Could you check a few things on this model? Use its own coordinates, in mm. Face numbers are marked on the shaded views. Give positions to 0.01 mm unless a question says otherwise; leave off trailing zeros. Write each loop counter-clockwise with the first axis right and the second up, starting at its lowest first coordinate (ties: lowest second). Pieces come first, ordered by that corner, then holes. Notation, with made-up numbers: (58, -15.75) - (108, -15.75) arc R27 cw to (108, 1.25) - close; hole circle Ø1 at (2, 20.25). An arc over 180 degrees is marked (long way). Answer in a Markdown table with one row per item.
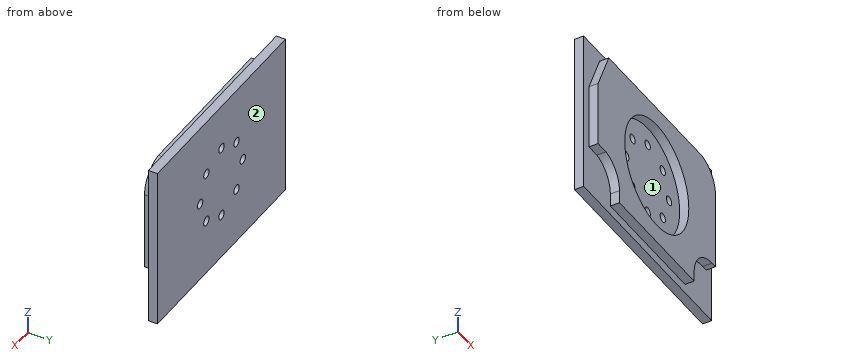
from build123d import *

# Parameters (mm, degrees)
F0_W     = 120
F0_H     = 90
F1_DEPTH = 5
F3_D     = 5
F4_R     = 2.5
F5_DEPTH = 5
F6_R     = 30
F7_DEPTH = 5


with BuildPart() as f1:
    # F0 (on Front) → F1 (new body)
    with BuildSketch(Plane.XZ):
        with Locations((-60, 45)):
            Rectangle(F0_W, F0_H)
    extrude(amount=F1_DEPTH)

    # F3 (through all)
    with Locations(Plane.XZ.offset(5)):
        with Locations((-74.144270925, 59.14), (-60, 65), (-45.86, 59.144270925), (-40, 45), (-45.855729075, 30.86), (-60, 25), (-80, 45), (-74.144270925, 30.86)):
            Hole(F3_D / 2)

    # F4 (on face) → F5 (join)
    with BuildSketch(Plane.XZ.offset(5)):
        with BuildLine():
            Line((-5, 27), (-5, 70.1358293132))
            ThreePointArc((-5, 70.1358293132), (-8.7037424203, 80.0046977738), (-17.985941959, 85))
            Line((-17.985941959, 85), (-105, 85))
            Line((-105, 85), (-115, 63))
            Line((-115, 63), (-115, 27))
            Line((-115, 27), (-107.5818091631, 27))
            ThreePointArc((-107.5818091631, 27), (-98.5703704663, 21.9102960199), (-95, 12.1962047746))
            Line((-95, 12.1962047746), (-95, 5))
            Line((-95, 5), (-25, 5))
            Line((-25, 5), (-25, 10.2326651871))
            ThreePointArc((-25, 10.2326651871), (-20.0889613357, 22.0889613357), (-8.2326651871, 27))
            Line((-8.2326651871, 27), (-5, 27))
        make_face()
        with Locations((-74.144270925, 30.86)):
            Circle(F4_R, mode=Mode.SUBTRACT)
        with Locations((-60, 25)):
            Circle(F4_R, mode=Mode.SUBTRACT)
        with Locations((-45.855729075, 30.86)):
            Circle(F4_R, mode=Mode.SUBTRACT)
        with Locations((-80, 45)):
            Circle(F4_R, mode=Mode.SUBTRACT)
        with Locations((-74.144270925, 59.14)):
            Circle(F4_R, mode=Mode.SUBTRACT)
        with Locations((-40, 45)):
            Circle(F4_R, mode=Mode.SUBTRACT)
        with Locations((-45.86, 59.144270925)):
            Circle(F4_R, mode=Mode.SUBTRACT)
        with Locations((-60, 65)):
            Circle(F4_R, mode=Mode.SUBTRACT)
    extrude(amount=F5_DEPTH)

    # F6 (on face) → F7 (cut)
    with BuildSketch(Plane.XZ.offset(10)):
        with Locations((-60, 45)):
            Circle(F6_R)
    extrude(amount=-F7_DEPTH, mode=Mode.SUBTRACT)


solid = f1.part
1) If I drill on line 1 (Z direction, x = -45.86, y = -2.1); line 2 (Z direction, x = -60, y = -6.8); line 3 (Z direction, x = -26, y = -7), over which ranges is the centre line in solid material (lowest first)?
Check values:
| item | result |
|---|---|
| line 1 | z = 0 to 28.36, 33.36 to 56.64, 61.64 to 90 |
| line 2 | z = 5 to 15, 75 to 85 |
| line 3 | z = 5 to 85 |
2) Imagine slicing it at C-C (z = 45). List the corners of the cut face in (x, y) for me.
Check values:
| item | result |
|---|---|
| outline | (-120, -5) - (-115, -5) - (-115, -10) - (-90, -10) - (-90, -5) - (-82.5, -5) - (-82.5, 0) - (-120, 0) - close; (-77.5, -5) - (-42.5, -5) - (-42.5, 0) - (-77.5, 0) - close; (-37.5, -5) - (-30, -5) - (-30, -10) - (-5, -10) - (-5, -5) - (0, -5) - (0, 0) - (-37.5, 0) - close |
3) We'd pull the mould along Z, two halves only. Please class the marked faces 1 and 2: +Z half, -Z half, draft (parallel to the pull), parting line (faces both ways), or undercut.
Check values:
| item | result |
|---|---|
| face 1 | undercut |
| face 2 | draft |
4) Imagine slicing it at B-B (x = -60). List the corners of the cut face in (y, z) for me, then the cut area to 3 significant figures.
Check values:
| item | result |
|---|---|
| outline | (-10, 5) - (-5, 5) - (-5, 0) - (0, 0) - (0, 22.5) - (-5, 22.5) - (-5, 15) - (-10, 15) - close; (-10, 75) - (-5, 75) - (-5, 67.5) - (0, 67.5) - (0, 90) - (-5, 90) - (-5, 85) - (-10, 85) - close; (-5, 27.5) - (0, 27.5) - (0, 62.5) - (-5, 62.5) - close |
| area | 500 mm2 |
5) Imagine slicing it at A-A (y = -7.5). List the corners of the cut face in (x, z) for me.
Check values:
| item | result |
|---|---|
| outline | (-115, 27) - (-107.58, 27) arc R15 cw to (-95, 12.2) - (-95, 5) - (-25, 5) - (-25, 10.23) arc R16.77 cw to (-8.23, 27) - (-5, 27) - (-5, 70.14) arc R15 ccw to (-17.99, 85) - (-105, 85) - (-115, 63) - close; hole circle Ø60 at (-60, 45) |
6) Will these pins go through, and if not, where does the flat tip stop? P1, Ø6.5, axis at x = -45.86, z = 59.14, coming from the -Y side; P2, Ø2.5, axis at x = -41.5, y = -7, coming from the +Z side; P3, Ø3, axis at x = -29.5, z = 54, coming from the +Y side; P4, Ø3, axis at x = -12, y = -8.5, coming from the +Z side.
Check values:
| item | result |
|---|---|
| P1 | stops at y = -5 |
| P2 | stops at z = 85 |
| P3 | stops at y = 0 |
| P4 | stops at z = 83.65 |
7) Imagine slicing it at D-D (z = 65). List the corners of the cut face in (x, y) for me.
Check values:
| item | result |
|---|---|
| outline | (-120, -5) - (-114.09, -5) - (-114.09, -10) - (-82.36, -10) - (-82.36, -5) - (-62.5, -5) - (-62.5, 0) - (-120, 0) - close; (-57.5, -5) - (-37.64, -5) - (-37.64, -10) - (-5, -10) - (-5, -5) - (0, -5) - (0, 0) - (-57.5, 0) - close |
